Part print with two shaded views. Sizes in mm from the minimum x, y, z corner. Coordinates: 2 decimals unless noted, no trailing zeros. Write each loop counter-clockwise with the first axis right and the second up, starting at its lowest first coordinate (ties: lowest second). Pieces come first, ordered by that corner, then holes.
Q1. Band-saw the part on C-C, the plane x = 22.86. State how many separate pieces and enclosed holes the cut face has, plus the area to 3 significant figures.
Q2. Drill centre lines: probe 1 along X at (y, z) = (26.5, 6) (1 decimal); probe 2 along X at (y, z) = (4, 5.25); probe 3 along Y at (x, z) = (47.5, 2.5) (1 decimal). Where is each one in solid material? Low to high.
Q3. Band-saw the part on A-A, the plane y = 3.81. Write the cut outline in (x, z).
Q4. Pin check, flat tips, straight feed: P1, Ø21.5, axis at x = 47.47, y = 27.58, coming from the -Z side; P2, Ø5, axis at x = 54.61, y = 3.81, coming from the +Z side; P3, Ø3, axis at y = 37.5, z = 2, coming from the -X side (1 decimal). Stop position of each tip, or through.
Q5. Pull direction Y, two halves, no side cores. Call the marked faces 1, 2, 3 and 4: released by +Y, released by -Y, zero draft, split by the parting line, or undercut.
Q6. Band-saw the part on B-B, the plane x = 67.31. Write the cut outline in (y, z).
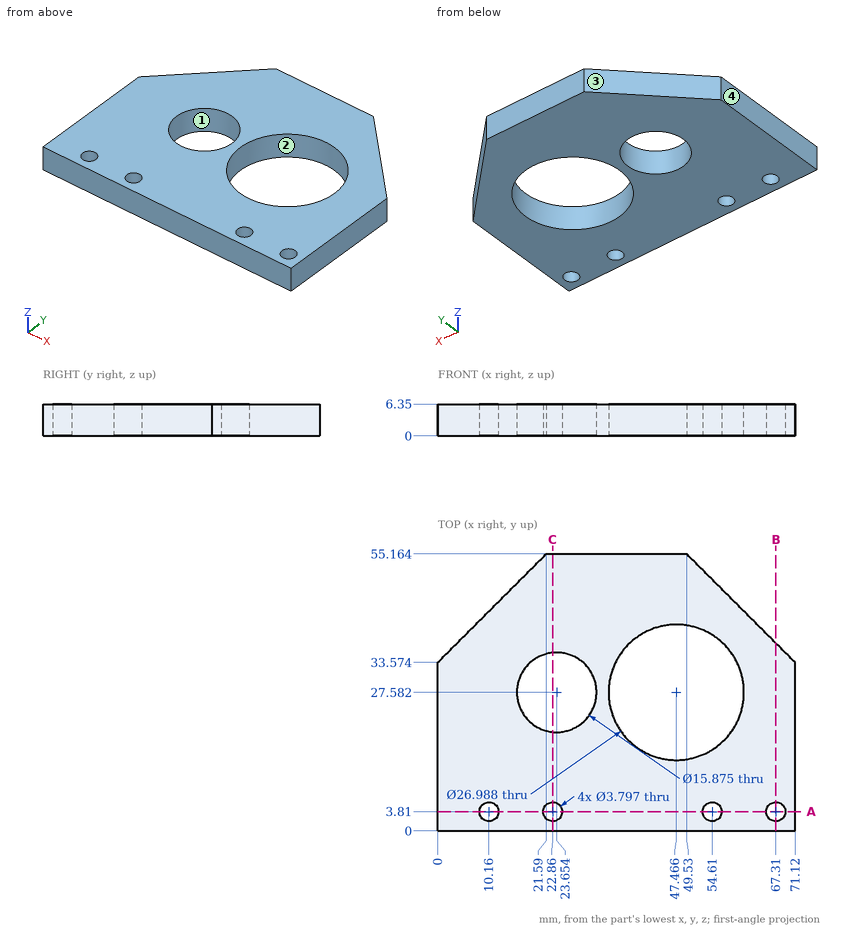
Answer sheet:
1. separate pieces: 3
1. enclosed holes: 0
1. area: 226 mm2
2. probe 1: x = 0 to 15.8, 31.5 to 34, 60.9 to 71.1
2. probe 2: x = 0 to 8.27, 12.05 to 20.97, 24.75 to 52.72, 56.5 to 65.42, 69.2 to 71.12
2. probe 3: y = 0 to 14.1, 41.1 to 55.2
3. outline: (0, 0) - (8.26, 0) - (8.26, 6.35) - (0, 6.35) - close; (12.06, 0) - (20.96, 0) - (20.96, 6.35) - (12.06, 6.35) - close; (24.76, 0) - (52.71, 0) - (52.71, 6.35) - (24.76, 6.35) - close; (56.51, 0) - (65.41, 0) - (65.41, 6.35) - (56.51, 6.35) - close; (69.21, 0) - (71.12, 0) - (71.12, 6.35) - (69.21, 6.35) - close
4. P1: passes through
4. P2: stops at z = 6.35
4. P3: stops at x = 2.4
5. face 1: undercut
5. face 2: undercut
5. face 3: released by +Y
5. face 4: zero draft
6. outline: (0, 0) - (1.91, 0) - (1.91, 6.35) - (0, 6.35) - close; (5.71, 0) - (37.38, 0) - (37.38, 6.35) - (5.71, 6.35) - close
